Part model, mm, in its own coordinate system. Face numbers are marked on the shaded views. A direction names the side the tool comes from. Coordinates: 2 decimals unless noted, no trailing zeros. Loops run counter-clockwise (first coordinate to the right, second up) from the corner with the lowest first, then second, coordinate; pieces in that order, holes last. Notation, with made-up numbers: M 43,39 L 87,39 A30 cw 87,67 Z; hole C 6,-34 d4. An arc over 180 degrees is marked long. Use a Markdown table: item, result. Add a question column.
1) Pin check, flat tips, straight feed: pin 1 Ø1 at (x, z) = (1.5, -3.5) entering from -Y; pin 2 Ø0.6 at (x, y) = (-4, 1) entering from -Z; pin 3 Ø0.6 at (y, z) = (1.5, -4) entering from -X. Stop position of each tip, or through.
2) Band-saw the part on A-A (y = -0.45). List the corners of the cut face in (x, z) (3 decimals).
3) Band-saw the part on C-C (x = -3). List the corners of the cut face in (y, z).
4) Wall check: probe 1 along X at (y, z) = (-0.4, 0) (3 decimals); probe 2 along Y at (x, z) = (-2.75, -0.5); probe 3 along Z at (x, y) = (-3.25, 0.4). Give the ranges that are in metal, low to high. Write a range as from..to.
5) Tool access for the marked faces 4, 5 and 6: list every direction of +Z, -Z, +X, -X, +Y, -Y with a clear straight run to the whole face (end or side of a thin tool).
6) Band-saw the part on B-B (z = 0). List the corners of the cut face in (x, y) (3 decimals), plus the area to 3 significant figures.
7) Pull direction X, two halves, no side cores. Call the marked faces 1, 2 and 3: released by +X, released by -X, zero draft, split by the parting line, or undercut.
8) Band-saw the part on D-D (z = 4). List the corners of the cut face in (x, y), plus the area to 3 significant figures.
from build123d import *

# Parameters (mm, degrees)
EXTRUDE_1_DEPTH = 2
SKETCH_2_R      = 2.575
SKETCH_2_R_2    = 0.85
EXTRUDE_2_DEPTH = 1


with BuildPart() as part:
    # ｽｹｯﾁ1 → ﾎﾞｽ - 押し出し1 (new body)
    with BuildSketch(Plane(origin=(0, 0, 0), x_dir=(1, 0, 0), z_dir=(0, 1, 0))):
        with BuildLine():
            Line((2.65, 4.705050478), (2.65, 2.65))
            Line((2.65, 2.65), (4.705050478, 2.65))
            ThreePointArc((4.705050478, 2.65), (5.4, 0), (4.705050478, -2.65))
            Line((4.705050478, -2.65), (2.65, -2.65))
            Line((2.65, -2.65), (2.65, -4.705050478))
            ThreePointArc((2.65, -4.705050478), (0, -5.4), (-2.65, -4.705050478))
            Line((-2.65, -4.705050478), (-2.65, -2.65))
            Line((-2.65, -2.65), (-4.705050478, -2.65))
            ThreePointArc((-4.705050478, -2.65), (-5.4, 0), (-4.705050478, 2.65))
            Line((-4.705050478, 2.65), (-2.65, 2.65))
            Line((-2.65, 2.65), (-2.65, 4.705050478))
            ThreePointArc((-2.65, 4.705050478), (0, 5.4), (2.65, 4.705050478))
        make_face()
        Polygon((0, 1.675), (0.437016815, 2.056002469), (0.681283877, 1.530188642), (1.235486269, 1.700500964), (1.244767583, 1.120793766), (1.820328922, 1.050967393), (1.593019665, 0.517603466), (2.090420168, 0.219712013), (1.665824175, -0.175085176), (1.999058776, -0.64953357), (1.450592551, -0.8375), (1.56204196, -1.406468898), (0.984540298, -1.355103466), (0.854933899, -1.920212977), (0.348252082, -1.638397231), (0, -2.101934787), (-0.348252082, -1.638397231), (-0.854933899, -1.920212977), (-0.984540298, -1.355103466), (-1.56204196, -1.406468898), (-1.450592551, -0.8375), (-1.999058776, -0.64953357), (-1.665824175, -0.175085176), (-2.090420168, 0.219712013), (-1.593019665, 0.517603466), (-1.820328922, 1.050967393), (-1.244767583, 1.120793766), (-1.235486269, 1.700500964), (-0.681283877, 1.530188642), (-0.437016815, 2.056002469), align=None, mode=Mode.SUBTRACT)
    extrude(amount=EXTRUDE_1_DEPTH)

    # ｽｹｯﾁ2 → ﾎﾞｽ - 押し出し2 (add)
    with BuildSketch(Plane.XZ):
        with Locations(Location((0, 0, 0), (0, 0, 90))):
            Circle(SKETCH_2_R)
        with Locations(Location((0, 0, 0), (0, 0, 270))):
            Circle(SKETCH_2_R_2, mode=Mode.SUBTRACT)
    extrude(amount=EXTRUDE_2_DEPTH)


solid = part.part
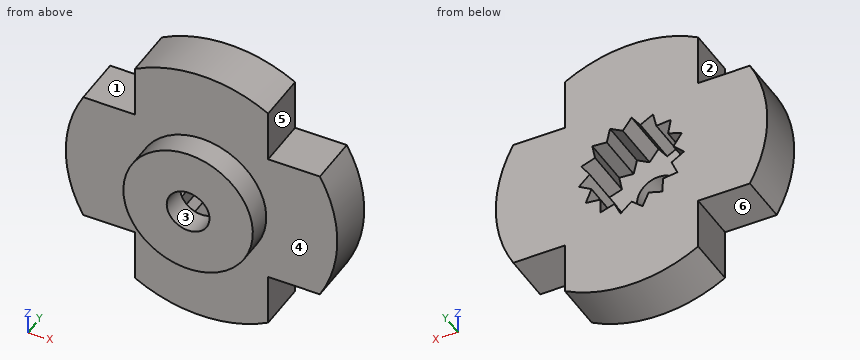
Entries:
| question | item | result |
|---|---|---|
| 1 | pin 1 | y = 0 |
| 1 | pin 2 | z = -2.65 |
| 1 | pin 3 | x = -2.65 |
| 2 | outline | C 0,0 d5.15; hole C 0,0 d1.7 |
| 3 | outline | M 0,-2.65 L 2,-2.65 L 2,2.65 L 0,2.65 Z |
| 4 | probe 1 | -2.575..-0.85, 0.85..2.575 |
| 4 | probe 2 | 0..2 |
| 4 | probe 3 | -2.65..2.65 |
| 5 | face 4 | -Y |
| 5 | face 5 | +Z, +X, +Y, -Y |
| 5 | face 6 | -Z, -X, +Y, -Y |
| 6 | outline | M -5.4,0 L -2.575,0 L -2.575,-1 L -0.85,-1 L -0.85,0 L -1.854,0 L -1.854,2 L -5.4,2 Z; M 0.85,-1 L 2.575,-1 L 2.575,0 L 5.4,0 L 5.4,2 L 1.854,2 L 1.854,0 L 0.85,0 Z |
| 6 | area | 17.6 mm2 |
| 7 | face 1 | zero draft |
| 7 | face 2 | released by -X |
| 7 | face 3 | undercut |
| 8 | outline | M -2.65,0 L 2.65,0 L 2.65,2 L -2.65,2 Z |
| 8 | area | 10.6 mm2 |
